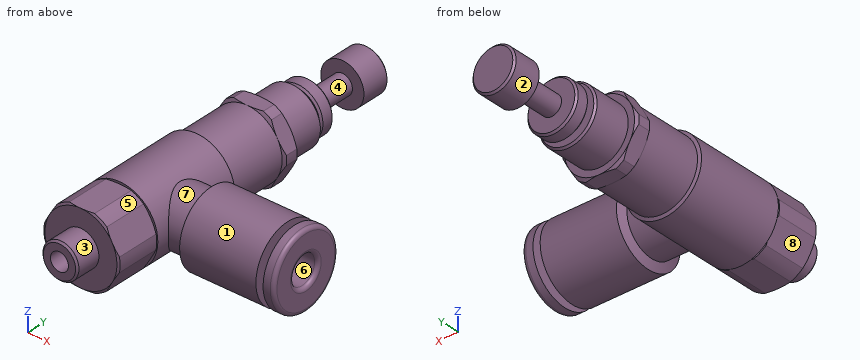
```python
from build123d import *

# Parameters (mm, degrees)
NUT_TOP_DEPTH               = 2.2
NUT_BOT_DEPTH               = 6.3
NUT_ROUNDS_DEPTH            = 25.203994161
NUT_ROUNDS_DEPTH_BACK       = 25.203994161
NUT_ROUNDS_SKETCH_OUTSIDE_W = 20.176
NUT_ROUNDS_SKETCH_OUTSIDE_H = 19.228
NUT_ROUNDS_SKETCH_OUTSIDE_R = 5.3
THREADS_SKETCH_R            = 2.5
THREADS_DEPTH               = 3.5
THREADS_MGT_SKETCH_R        = 4
THREADS_MGT_DEPTH           = 5.3
LOC_SPACER_SKETCH_R         = 2
LOC_SPACER_DEPTH            = 0.5
LOC_ADJUSTER_SKETCH_R       = 3.5
LOC_ADJUSTER_DEPTH          = 2
TUBE_SKETCH_R               = 2
TUBE_DEPTH                  = 13
TUBE_ROUDS_R                = 0.5
PROFILE_PORT_R              = 1.25
CHAM_SIZE                   = 0.25


with BuildPart() as part:
    # MBody_Sketch → MBody (revolve)
    with BuildSketch(Plane.XY, mode=Mode.PRIVATE) as mbody_sk:
        Polygon((0, 17.2), (-4.875, 17.2), (-4.875, 6.95468735), (-5.3, 6.8), (-5.3, -5.7), (0, -5.7), align=None)
    revolve(mbody_sk.sketch.rotate(Axis((0, 0, 0), (0, 1, 0)), 270), axis=Axis((0, 0, 0), (0, 1, 0)))

    # Nut Top_Sketch → Nut Top (add)
    with BuildSketch(Plane(origin=(0, 17.2, 0), x_dir=(-1, 0, 0), z_dir=(0, 1, 0))):
        Polygon((-2.814582562, 4.875), (-5.629165125, 0), (-2.814582562, -4.875), (2.814582562, -4.875), (5.629165125, 0), (2.814582562, 4.875), align=None)
    extrude(amount=-NUT_TOP_DEPTH)

    # Nut Cham Top_Sketch → Nut Cham Top (revolve, cut)
    with BuildSketch(Plane.XY):
        Polygon((5.629165125, 17.2), (4.875, 17.2), (5.629165125, 16.764582562), align=None)
        Polygon((5.629165125, 15.435417438), (5.629165125, 15), (4.875, 15), align=None)
    revolve(axis=Axis((0, 0, 0), (0, 1, 0)), mode=Mode.SUBTRACT)

    # Nut Bot_Sketch → Nut Bot (add)
    with BuildSketch(Plane.XZ.offset(5.7)):
        Polygon((2.886751346, -5), (5.773502692, 0), (2.886751346, 5), (-2.886751346, 5), (-5.773502692, 0), (-2.886751346, -5), align=None)
    extrude(amount=NUT_BOT_DEPTH)

    # Nut Cham Bot_Sketch → Nut Cham Bot (revolve, cut)
    with BuildSketch(Plane.XY):
        Polygon((5.773502692, -5.7), (5, -5.7), (5.773502692, -6.146581987), align=None)
        Polygon((5.773502692, -11.553418013), (5.773502692, -12), (5, -12), align=None)
    revolve(axis=Axis((0, -2.270147765, 0), (0, -1, 0)), mode=Mode.SUBTRACT)

    # Nut Rounds_Sketch outside → Nut Rounds (cut, two sides: drawn at the far end of the back side and taken through both)
    with BuildSketch(Plane(origin=(0, -5.7, 0), x_dir=(-1, 0, 0), z_dir=(0, 1, 0)).offset(-NUT_ROUNDS_DEPTH_BACK)):
        Rectangle(NUT_ROUNDS_SKETCH_OUTSIDE_W, NUT_ROUNDS_SKETCH_OUTSIDE_H)
        with Locations(Location((0, 0, 0), (0, 0, 270))):
            Circle(NUT_ROUNDS_SKETCH_OUTSIDE_R, mode=Mode.SUBTRACT)
    extrude(amount=NUT_ROUNDS_DEPTH + NUT_ROUNDS_DEPTH_BACK, mode=Mode.SUBTRACT)

    # Threads_Sketch → Threads (add)
    with BuildSketch(Plane(origin=(0, -12, 0), x_dir=(-1, 0, 0), z_dir=(0, 1, 0))):
        with Locations(Location((0, 0, 0), (0, 0, 90))):
            Circle(THREADS_SKETCH_R)
    extrude(amount=-THREADS_DEPTH)

    # Threads MGT_Sketch → Threads MGT (add)
    with BuildSketch(Plane(origin=(0, 17.2, 0), x_dir=(-1, 0, 0), z_dir=(0, 1, 0))):
        with Locations(Location((0, 0, 0), (0, 0, 270))):
            Circle(THREADS_MGT_SKETCH_R)
    extrude(amount=THREADS_MGT_DEPTH)

    # Adjuster_Sketch → Adjuster (revolve)
    with BuildSketch(Plane.XY, mode=Mode.PRIVATE) as adjuster_sk:
        Polygon((0, 17.2), (0, 34.5), (3, 34.5), (3, 30.5), (1.4, 30.5), (1.4, 17.2), align=None)
    revolve(adjuster_sk.sketch.rotate(Axis((0, 0, 0), (0, 1, 0)), 90), axis=Axis((0, 0, 0), (0, 1, 0)))

    # Loc Spacer_Sketch → Loc Spacer (add)
    with BuildSketch(Plane(origin=(0, 22.5, 0), x_dir=(-1, 0, 0), z_dir=(0, 1, 0))):
        with Locations(Location((0, 0, 0), (0, 0, 90))):
            Circle(LOC_SPACER_SKETCH_R)
    extrude(amount=LOC_SPACER_DEPTH)

    # Loc Adjuster_Sketch → Loc Adjuster (add)
    with BuildSketch(Plane(origin=(0, 23, 0), x_dir=(-1, 0, 0), z_dir=(0, 1, 0))):
        with Locations(Location((0, 0, 0), (0, 0, 90))):
            Circle(LOC_ADJUSTER_SKETCH_R)
    extrude(amount=LOC_ADJUSTER_DEPTH)

    # RBody_Sketch → RBody (revolve)
    with BuildSketch(Plane.XY, mode=Mode.PRIVATE) as rbody_sk:
        Polygon((0, 0), (0, 4), (7.463235719, 4), (7.9, 5.2), (18.5, 5.2), (18.5, 0), align=None)
    revolve(rbody_sk.sketch.rotate(Axis((0, 0, 0), (1, 0, 0)), 90), axis=Axis((0, 0, 0), (1, 0, 0)))

    # Release_Sketch → Release (revolve)
    with BuildSketch(Plane.XY, mode=Mode.PRIVATE) as release_sk:
        Polygon((18.5, 0), (18.5, 2.75), (19.5, 2.75), (19.5, 5.2), (21, 5.2), (21, 0), align=None)
    revolve(release_sk.sketch.rotate(Axis((0, 0, 0), (1, 0, 0)), 90), axis=Axis((0, 0, 0), (1, 0, 0)))

    # Tube_Sketch → Tube (cut)
    with BuildSketch(Plane(origin=(21, 0, 0), x_dir=(0, 0, -1), z_dir=(1, 0, 0))):
        Circle(TUBE_SKETCH_R)
    extrude(amount=-TUBE_DEPTH, mode=Mode.SUBTRACT)

    # Tube Rouds
    tube_rouds_edges = [part.edges().sort_by_distance(p)[0] for p in [
        (21, 0, -5.2),
        (21, 0, 2),
    ]]
    fillet(tube_rouds_edges, radius=TUBE_ROUDS_R)

    # Port: sweep along a path in Path Port
    with BuildLine(Plane.XY) as port_path:
        Line((21, 0), (3, 0))
        ThreePointArc((3, 0), (0.878679656, -0.878679656), (0, -3))
        Line((0, -3), (0, -15.5))
    # Profile Port → Port (sweep, cut)
    with BuildSketch(Plane(origin=(21, 0, 0), x_dir=(0, 0, -1), z_dir=(1, 0, 0))):
        Circle(PROFILE_PORT_R)
    sweep(path=port_path.line, mode=Mode.SUBTRACT)

    # Cham
    cham_edges = [part.edges().sort_by_distance(p)[0] for p in [
        (0, -15.5, -2.5),
        (0, 22.5, 4),
        (0, 34.5, 3),
        (0, 23, -3.5),
        (0, 25, -3.5),
    ]]
    chamfer(cham_edges, length=CHAM_SIZE)


solid = part.part
```
Check sheet for the modelled part. Datum: model origin and axes. Units: mm. Face numbers are marked on the shaded views. A direction names the side the tool comes from. Coordinates: 2 decimals unless noted, no trailing zeros. Order: outer loops, then holes, each group sorted by start corner. A loop starts at its lowest first (then second) coordinate and runs counter-clockwise, first axis right, second up. Notation, with made-up numbers: M 9.25,41.25 L 65.25,41.25 A28 cw 65.25,65.25 Z; hole C -6,-14.75 d7. An arc over 180 degrees is marked long. One line per question, with ' | ' between items. Start each with the question number.
Item 1: Material ranges on line 1 (Y direction, x = 11.5, z = 0); line 2 (Y direction, x = 2.5, z = 2); line 3 (X direction, y = -2, z = 4.25), recorded low to high.
Item 2: Mould release check, pull along Z, two halves, no side actions. Record for the marked faces 5, 6, 7 and 8: pulls with the +Z half, pulls with the -Z half, needs draft (parallel to the pull), parting line crosses it, or undercut.
Item 3: Gauge pin test, flat ends, axial feed: P1, Ø3, axis at y = -2, z = 0.5, coming from the +X side; P2, Ø6, axis at y = 23, z = 3.5, coming from the -X side; P3, Ø3, axis at x = 0, y = -8, coming from the +Z side; P4, Ø3, axis at x = -1, y = -7.5, coming from the -Z side. Record the tip position at first contact, or that the pin passes through.
Item 4: Access from +Z, -Z, +X, -X, +Y, -Y to the whole of each face (thin tool, end or side, straight path). Record for the marked faces 1, 2, 3 and 4.
Item 5: Sectioned sample at C-C on y = 26. Record the cut outline in (x, z).
Item 6: Sectioned sample at B-B on y = 10. Record the cut outline in (x, z) (3 decimals), and give its area (3 significant figures).
Item 7: Sectioned sample at A-A on x = 17.25. Record the cut outline in (y, z).
Answer below:
1) line 1: y = -5.2 to -2, 2 to 5.2 | line 2: y = -12 to 22.5, 23 to 25 | line 3: x = -3.17 to 3.17, 7.72 to 18.5, 19.5 to 21
2) face 5: pulls with the +Z half | face 6: undercut | face 7: parting line crosses it | face 8: pulls with the -Z half
3) P1: stops at x = 21 | P2: stops at x = -3.96 | P3: stops at z = 5 | P4: stops at z = -5
4) face 1: +X | face 2: +Y | face 3: -Y | face 4: none
5) outline: C 0,0 d2.8
6) outline: C 0,0 d9.75 | area: 74.7 mm^2
7) outline: C 0,0 d10.4; hole C 0,0 d4
